Read the model definition and answer for the solid it produces. Units are mm, in the model's axes. A direction names the side the tool comes from. Give positions to 0.01 mm unless a question says otherwise; leave off trailing zeros. Order: outer loops, then holes, each group sorted by start corner. A loop starts at its lowest first (then second) coordinate and runs counter-clockwise, first axis right, second up. Notation, with made-up numbers: (-5.75, 24.25) -> (52.25, 24.25) arc R14 cw to (52.25, 43.25) -> close; hole circle Ø7 at (11.25, 55.25). An arc over 180 degrees is marked (long way). One line per item, written item: value. Start each with the question number.
from build123d import *

# Parameters (mm, degrees)
F0_R     = 12.5
F0_R_2   = 10.5
F1_DEPTH = 25
F3_DEPTH = 3
F5_DEPTH = 3


with BuildPart() as f1:
    # F0 (on Top) → F1 (new body)
    with BuildSketch(Plane.XY):
        Circle(F0_R)
        Circle(F0_R_2, mode=Mode.SUBTRACT)
    extrude(amount=F1_DEPTH)

    # F2 (on face) → F3 (join)
    with BuildSketch(Plane.XY.offset(25)):
        with BuildLine():
            ThreePointArc((1.801071, 12.369565), (0, 12.5), (-1.801071, 12.369565))
            ThreePointArc((-1.801071, 12.369565), (0, 9.5), (1.801071, 12.369565))
        make_face()
        with BuildLine():
            ThreePointArc((1.801071, -12.369565), (0, -9.5), (-1.801071, -12.369565))
            ThreePointArc((-1.801071, -12.369565), (0, -12.5), (1.801071, -12.369565))
        make_face()
    extrude(amount=-F3_DEPTH)

    # F4 (on face) → F5 (join)
    with BuildSketch(Plane(origin=(0, 0, 0), x_dir=(1, 0, 0), z_dir=(0, 0, -1))):
        with BuildLine():
            ThreePointArc((1.801071, 12.369565), (0, 12.5), (-1.801071, 12.369565))
            ThreePointArc((-1.801071, 12.369565), (0, 9.5), (1.801071, 12.369565))
        make_face()
        with BuildLine():
            ThreePointArc((1.801071, -12.369565), (0, -9.5), (-1.801071, -12.369565))
            ThreePointArc((-1.801071, -12.369565), (0, -12.5), (1.801071, -12.369565))
        make_face()
    extrude(amount=-F5_DEPTH)


solid = f1.part
Item 1: For a pull along Z with two mould halves and no side action, classify faces 4 (the flat face through (0, 10, 3)), 5 (the flat face through (-1, 10, 0)), 6 (the flat face through (0, 10, 22)), 7 (the cylindrical face through (0, -9.5, 23.5)) as +Z half, -Z half, draft (parallel to the pull), parting line (faces both ways), or undercut.
Item 2: Flat-ended cylindrical pins translate along their axes: pin 1 (5 mm diameter, centred on x = 0.5, y = -6.5, fed in from +Z); pin 2 (8 mm diameter, centred on x = 8, z = 7.5, fed in from -Y); pin 3 (5 mm diameter, centred on y = -3.5, z = 15.5, fed in from -X); pin 4 (5 mm diameter, centred on y = -7.5, z = 19, fed in from -X). Find the tip coordinate at first contact, or state that the pin passes through.
Item 3: Find section A-A on y = 0. Write down the section's boundary in (x, z).
Item 4: Find section C-C on z = 15.5. Write down the section's boundary in (x, y).
Item 5: A tool of negligible diameter and unlimited length cuts with its end or side. For faces 1 (the flat face through (0, -10, 22)), 2 (the cylindrical face through (0, -12.5, 23.5)), 3 (the cylindrical face through (0, -9.5, 1.5)), from which of +Z, -Z, +X, -X, +Y, -Y can it reach the whole face along a straight path? Write none if from no direction.
Item 6: Find the intervals of material crossed by line 1 (X direction, y = 0, z = 15.5); line 2 (Y direction, x = 7, z = 11), in increasing order. Write a range as from..to.
Item 7: Find section B-B on x = -9. Write down the section's boundary in (y, z), then the cut area to 3 significant figures.
Item 8: Find section D-D on x = 0. Write down the section's boundary in (y, z), then the cut area to 3 significant figures.
Checks:
1. face 4: undercut
1. face 5: -Z half
1. face 6: undercut
1. face 7: draft
2. pin 1: through
2. pin 2: y = -11.84
2. pin 3: x = -12.46
2. pin 4: x = -11.46
3. outline: (-12.5, 0) -> (-10.5, 0) -> (-10.5, 25) -> (-12.5, 25) -> close; (10.5, 0) -> (12.5, 0) -> (12.5, 25) -> (10.5, 25) -> close
4. outline: circle Ø25 at (0, 0); hole circle Ø21 at (0, 0)
5. face 1: none
5. face 2: +Z, -Z, -Y
5. face 3: +Z, -Z
6. line 1: -12.5..-10.5, 10.5..12.5
6. line 2: -10.36..-7.83, 7.83..10.36
7. outline: (-8.67, 0) -> (-5.41, 0) -> (-5.41, 25) -> (-8.67, 25) -> close; (5.41, 0) -> (8.67, 0) -> (8.67, 25) -> (5.41, 25) -> close
7. area: 163 mm2
8. outline: (-12.5, 0) -> (-9.5, 0) -> (-9.5, 3) -> (-10.5, 3) -> (-10.5, 22) -> (-9.5, 22) -> (-9.5, 25) -> (-12.5, 25) -> close; (9.5, 0) -> (12.5, 0) -> (12.5, 25) -> (9.5, 25) -> (9.5, 22) -> (10.5, 22) -> (10.5, 3) -> (9.5, 3) -> close
8. area: 112 mm2
